from build123d import *

# Parameters (mm, degrees)
CROQUIS1_W                                           = 177.5
CROQUIS1_H                                           = 250
CROQUIS1_R                                           = 2
CROQUIS1_R_2                                         = 3.4
CROQUIS1_R_3                                         = 3
CROQUIS1_R_4                                         = 4.5
SALIENTE_EXTRUIR1_DEPTH                              = 7
SALIENTE_EXTRUIR2_DEPTH                              = 70
REDONDEO1_R                                          = 10
CROQUIS4_W                                           = 10
CROQUIS4_H                                           = 65
SALIENTE_EXTRUIR3_DEPTH                              = 7
REDONDEO3_R                                          = 1
REDONDEO4_R                                          = 2.5
CROQUIS5_W                                           = 121
CROQUIS5_H                                           = 27.5
SALIENTE_EXTRUIR4_DEPTH                              = 20
AVELLANADO_PARA_TORNILLO_CON_CABEZA_OVAL_D           = 5.7912
AVELLANADO_PARA_TORNILLO_CON_CABEZA_OVAL_CSINK_D     = 11.1252
AVELLANADO_PARA_TORNILLO_CON_CABEZA_OVAL_CSINK_ANGLE = 82
CROQUIS15_R                                          = 1.5
CORTAR_EXTRUIR1_DEPTH                                = 5


with BuildPart() as part:
    # Croquis1 → Saliente-Extruir1 (new body)
    with BuildSketch(Plane(origin=(0, 4, 0), x_dir=(1, 0, 0), z_dir=(0, 1, 0))):
        with Locations((68.75, 0)):
            Rectangle(CROQUIS1_W, CROQUIS1_H)
        with Locations(Location((153.5, -20.15, 0), (0, 0, 90))):
            Circle(CROQUIS1_R, mode=Mode.SUBTRACT)
        with Locations(Location((144.6, 0, 0), (0, 0, 90))):
            Circle(CROQUIS1_R_2, mode=Mode.SUBTRACT)
        with Locations(Location((153.5, 20.15, 0), (0, 0, 90))):
            Circle(CROQUIS1_R, mode=Mode.SUBTRACT)
        with Locations(Location((37.5, 70, 0), (0, 0, 90))):
            Circle(CROQUIS1_R_3, mode=Mode.SUBTRACT)
        with Locations(Location((37.5, -70, 0), (0, 0, 90))):
            Circle(CROQUIS1_R_3, mode=Mode.SUBTRACT)
        with Locations(Location((7.5, -30.5, 0), (0, 0, 90))):
            Circle(CROQUIS1_R_4, mode=Mode.SUBTRACT)
        with Locations(Location((7.5, 30.5, 0), (0, 0, 90))):
            Circle(CROQUIS1_R_4, mode=Mode.SUBTRACT)
    extrude(amount=SALIENTE_EXTRUIR1_DEPTH)

    # Croquis3 → Saliente-Extruir2 (add)
    with BuildSketch(Plane(origin=(0, 11, 0), x_dir=(1, 0, 0), z_dir=(0, 1, 0))):
        with BuildLine():
            Line((-20, 125), (-20, -125))
            Line((-20, -125), (157.5, -125))
            Line((157.5, -125), (157.5, -33.65))
            ThreePointArc((157.5, -33.65), (153.721677477, -24.528322523), (144.6, -20.75))
            ThreePointArc((144.6, -20.75), (123.85, 0), (144.6, 20.75))
            ThreePointArc((144.6, 20.75), (153.721677477, 24.528322523), (157.5, 33.65))
            Line((157.5, 33.65), (157.5, 125))
            Line((157.5, 125), (-20, 125))
        make_face()
        with BuildLine():
            Line((149.5, 117), (-12, 117))
            Line((-12, 117), (-12, -117))
            Line((-12, -117), (149.5, -117))
            Line((149.5, -117), (149.5, -33.65))
            ThreePointArc((149.5, -33.65), (148.064823228, -30.185176772), (144.6, -28.75))
            ThreePointArc((144.6, -28.75), (115.85, 0), (144.6, 28.75))
            ThreePointArc((144.6, 28.75), (148.064823228, 30.185176772), (149.5, 33.65))
            Line((149.5, 33.65), (149.5, 117))
        make_face(mode=Mode.SUBTRACT)
    extrude(amount=SALIENTE_EXTRUIR2_DEPTH)

    # Redondeo1
    redondeo1_edges = [part.edges().sort_by_distance(p)[0] for p in [
        (-12, 46, 117),
        (149.5, 46, 117),
        (149.5, 46, -117),
        (-12, 46, -117),
        (-20, 42.5, -125),
        (157.5, 42.5, -125),
        (157.5, 42.5, 125),
        (-20, 42.5, 125),
    ]]
    fillet(redondeo1_edges, radius=REDONDEO1_R)

    # Croquis4 → Saliente-Extruir3 (add)
    with BuildSketch(Plane(origin=(0, 11, 0), x_dir=(1, 0, 0), z_dir=(0, 1, 0))):
        with Locations((162.5, 0)):
            Rectangle(CROQUIS4_W, CROQUIS4_H)
    extrude(amount=-SALIENTE_EXTRUIR3_DEPTH)

    # Redondeo3
    redondeo3_edges = [part.edges().sort_by_distance(p)[0] for p in [
        (157.5, 7.5, -32.5),
        (157.5, 7.5, 32.5),
    ]]
    fillet(redondeo3_edges, radius=REDONDEO3_R)

    # Redondeo4
    redondeo4_edges = [part.edges().sort_by_distance(p)[0] for p in [
        (167.5, 7.5, -32.5),
        (167.5, 7.5, 32.5),
    ]]
    fillet(redondeo4_edges, radius=REDONDEO4_R)

    # Croquis5 → Saliente-Extruir4 (add)
    with BuildSketch(Plane(origin=(0, 11, 0), x_dir=(1, 0, 0), z_dir=(0, 1, 0))):
        with Locations((48.5, -0.75)):
            Rectangle(CROQUIS5_W, CROQUIS5_H)
        with Locations((48.5, -93.25)):
            Rectangle(CROQUIS5_W, CROQUIS5_H)
    extrude(amount=SALIENTE_EXTRUIR4_DEPTH)

    # Avellanado para tornillo con cabeza ovalada de #121 (through all)
    with Locations(Plane(origin=(0, 4, 0), x_dir=(-1, 0, 0), z_dir=(0, -1, 0))):
        with Locations((-99.5, -93), (-20.5, -92.999999989), (-20.5, -0.999999991), (-99.5, -1)):
            CounterSinkHole(AVELLANADO_PARA_TORNILLO_CON_CABEZA_OVAL_D / 2, AVELLANADO_PARA_TORNILLO_CON_CABEZA_OVAL_CSINK_D / 2, counter_sink_angle=AVELLANADO_PARA_TORNILLO_CON_CABEZA_OVAL_CSINK_ANGLE)

    # Croquis15 → Cortar-Extruir1 (cut)
    with BuildSketch(Plane(origin=(0, 81, 0), x_dir=(1, 0, 0), z_dir=(0, 1, 0))):
        with Locations(Location((150.571067812, -118.071067812, 0), (0, 0, 270))):
            Circle(CROQUIS15_R)
        with Locations(Location((-13.071067812, -118.071067812, 0), (0, 0, 270))):
            Circle(CROQUIS15_R)
        with Locations(Location((-13.071067812, 118.071067812, 0), (0, 0, 90))):
            Circle(CROQUIS15_R)
        with Locations(Location((150.571067812, 118.071067812, 0), (0, 0, 90))):
            Circle(CROQUIS15_R)
    extrude(amount=-CORTAR_EXTRUIR1_DEPTH, mode=Mode.SUBTRACT)


solid = part.part
Work out the finished part from the listing and answer in its coordinate system (mm). A direction names the side the tool comes from. Give positions to 0.01 mm unless a question says otherwise; leave off trailing zeros. Write each loop counter-clockwise with the first axis right and the second up, starting at its lowest first coordinate (ties: lowest second). Pieces come first, ordered by that corner, then holes.
Q1. Straight lines are drawn through the part: L1, parallel to Z at x = 37, y = 8; L2, parallel to Z at x = 92.5, y = 15; L3, parallel to X at y = 19, z = 93. For each, find the intervals that lie inside material, in ascending order.
Answer:
L1: z = -125 to -72.96, -67.04 to 67.04, 72.96 to 125
L2: z = -125 to -117, -13 to 14.5, 79.5 to 107, 117 to 125
L3: x = -20 to 17.6, 23.4 to 96.6, 102.4 to 109, 149.5 to 157.5
Q2. The part is cut by section A-A on x = 37.5. Give the vertices of the cut face in (y, z), and give its area (3 significant figures).
Answer:
outline: (4, -125) - (81, -125) - (81, -117) - (11, -117) - (11, -73) - (4, -73) - close; (4, -67) - (11, -67) - (11, -13) - (31, -13) - (31, 14.5) - (11, 14.5) - (11, 67) - (4, 67) - close; (4, 73) - (11, 73) - (11, 79.5) - (31, 79.5) - (31, 107) - (11, 107) - (11, 117) - (81, 117) - (81, 125) - (4, 125) - close
area: 3,890 mm2
Q3. The part is cut by section D-D on x = 99.5. Give the vertices of the cut face in (y, z), and give its area (3 significant figures).
Answer:
outline: (4, -125) - (81, -125) - (81, -117) - (11, -117) - (11, -13) - (31, -13) - (31, -1.9) - (7.07, -1.9) - (4, -4.56) - close; (4, 6.56) - (7.07, 3.9) - (31, 3.9) - (31, 14.5) - (11, 14.5) - (11, 79.5) - (31, 79.5) - (31, 90.1) - (7.07, 90.1) - (4, 87.44) - close; (4, 98.56) - (7.07, 95.9) - (31, 95.9) - (31, 107) - (11, 107) - (11, 117) - (81, 117) - (81, 125) - (4, 125) - close
area: 3,640 mm2
Q4. For a pull along X with two mould halves and no side action, classify faces 5 (the face through (109, 21, 1)), 6 (the face through (157.5, 42, -74)), 7 (the face through (121, 81, -1)) as released by +X, released by -X, zero draft, split by the parting line, or undercut.
Answer:
face 5: undercut
face 6: released by +X
face 7: zero draft
Q5. The part is cut by section C-C on x = 7.5. Give the vertices of the cut face in (y, z), and give its area (3 significant figures).
Answer:
outline: (4, -125) - (81, -125) - (81, -117) - (11, -117) - (11, -35) - (4, -35) - close; (4, -26) - (11, -26) - (11, -13) - (31, -13) - (31, 14.5) - (11, 14.5) - (11, 26) - (4, 26) - close; (4, 35) - (11, 35) - (11, 79.5) - (31, 79.5) - (31, 107) - (11, 107) - (11, 117) - (81, 117) - (81, 125) - (4, 125) - close
area: 3,840 mm2
Q6. The part is cut by section B-B on z = -49. Give the vertices of the cut face in (x, y), and give its area (3 significant figures).
Answer:
outline: (-20, 4) - (157.5, 4) - (157.5, 81) - (149.5, 81) - (149.5, 11) - (-12, 11) - (-12, 81) - (-20, 81) - close
area: 2,360 mm2
Q7. A tool of negligible diameter and unlimited length cuts with its end or side. For faces 1 (the face through (70, 46, -117)), 2 (the face through (123.855, 45.51, 0.456)), 3 (the face through (147.92, 7.45, 0.74)), 4 (the face through (162, 8, 32.5)), from which of +Z, -Z, +X, -X, +Y, -Y can it reach the whole face along a straight path? Write none if from no direction.
Answer:
face 1: +Y
face 2: +X, +Y
face 3: +Y, -Y
face 4: +Z, +X, +Y, -Y
Q8. Given pin 1 (5 mm diameter, centred on x = 162.5, y = 6.5, fed in from -Z); pin 2 (22 mm diameter, centred on y = 24, z = 98.5, fed in from +X); pin 3 (4 mm diameter, centred on x = 66.5, z = -69.5, fed in from +Y), each flat-ended and moving along its own axis, determine where each tip first touches the part or whether it passes through.
Answer:
pin 1: stops at z = -32.5
pin 2: stops at x = 157.5
pin 3: stops at y = 11
